For this review, take the finished solid that the model builds, in its own axes (mm). A direction names the side the tool comes from. Give positions to 0.01 mm unless a question says otherwise; leave off trailing zeros. Loops run counter-clockwise (first coordinate to the right, second up) from the corner with the lowest first, then second, coordinate; pieces in that order, holes last.
```python
from build123d import *

# Parameters (mm, degrees)
BOSS_EXTRUDE1_DEPTH = 6.2
BOSS_EXTRUDE1_DRAFT = 6
SKETCH2_R           = 1.5
SKETCH2_R_2         = 2.5
CUT_EXTRUDE1_DEPTH  = 19.269236809
SHELL1_T            = -1.2


with BuildPart() as part:
    # Sketch1 → Boss-Extrude1 (with draft: the straight prism first)
    with BuildSketch(Plane(origin=(0, 0, 0), x_dir=(1, 0, 0), z_dir=(0, 1, 0))):
        with BuildLine():
            Line((-11.5, 11.5), (-11.5, 0))
            ThreePointArc((-11.5, 0), (0, -11.5), (11.5, 0))
            Line((11.5, 0), (11.5, 11.5))
            Line((11.5, 11.5), (-11.5, 11.5))
        make_face()
    extrude(amount=-BOSS_EXTRUDE1_DEPTH)
    # Boss-Extrude1: the draft: its side faces are tilted about the plane it starts from
    boss_extrude1_sides = [part.faces().sort_by_distance(p)[0] for p in [
        (11.5, -3.1, -5.75),
        (0, -3.1, -11.5),
        (-11.5, -3.1, -5.75),
        (0, -3.1, 11.5),
    ]]
    draft(boss_extrude1_sides, Plane(origin=(0, 0, 0), x_dir=(1, 0, 0), z_dir=(0, 1, 0)), BOSS_EXTRUDE1_DRAFT)

    # Sketch2 → Cut-Extrude1 (cut, through all)
    with BuildSketch(Plane(origin=(0, 0, 0), x_dir=(1, 0, 0), z_dir=(0, 1, 0))):
        with Locations(Location((-6, 3.464101615, 0), (0, 0, 270))):
            Circle(SKETCH2_R)
        with Locations(Location((6, 3.464101615, 0), (0, 0, 270))):
            Circle(SKETCH2_R)
        with Locations(Location((0, -6.92820323, 0), (0, 0, 270))):
            Circle(SKETCH2_R_2)
    extrude(amount=-CUT_EXTRUDE1_DEPTH, mode=Mode.SUBTRACT)

    # Shell1
    shell1_openings = [part.faces().sort_by_distance(p)[0] for p in [
        (0, -6.2, -1.388400602),
    ]]
    offset(amount=SHELL1_T, openings=shell1_openings)


solid = part.part
```
Q1. For probe 1 along Z at (x, y) = (-6.25, -4.5); probe 2 along Z at (x, y) = (8, -3.5); probe 3 along Z at (x, y) = (-3, -3.75), list the stretches that pass through material, from the lowest coordinate up.
Answers:
probe 1: z = -11.97 to -10.77, -6.15 to -4.94, -1.99 to -0.78, 8.77 to 10.21
probe 2: z = -11.87 to -10.66, -5.28 to -1.65, 7.05 to 8.77
probe 3: z = -11.89 to -10.69, 4.76 to 9.09, 10.26 to 11.51
Q2. Consider section B-B on x = 0. Give the boundary of the cut face in (y, z), plus the area to 3 significant figures.
Answers:
outline: (-6.2, -12.15) - (0, -11.5) - (0, 4.43) - (-6.2, 4.43) - (-6.2, 3.23) - (-1.2, 3.23) - (-1.2, -10.42) - (-6.2, -10.95) - close; (-6.2, 9.43) - (0, 9.43) - (0, 11.5) - (-6.2, 12.15) - (-6.2, 10.95) - (-3.19, 10.63) - (-6.2, 10.63) - close
area: 45.6 mm2
Q3. Machinability: for faces 1 (the cylindrical face through (6.451, -3.057, -2.033)), 2 (the flat face through (0.15, -3.67, -10.68)), which of the approach directions +Z, -Z, +X, -X, +Y, -Y give a long, thin tool a straight path to every point of the face, cutting with its end or side? Answer none if there is none.
Answers:
face 1: +Y, -Y
face 2: -Y
Q4. Mouldability with a two-part tool opening along Z and no side actions: class faces 3 (the flat face through (10.68, -3.67, -5.4)), 4 (the conical face through (-0.258, -2.368, 11.746)), 5 (the flat face through (0, -6.2, 4)) as +Z half, -Z half, draft (parallel to the pull), parting line (faces both ways), or undercut.
Answers:
face 3: undercut
face 4: +Z half
face 5: draft
Q5. Consider section A-A on y = -2.75. Give the boundary of the cut face in (x, z), plus the area to 3 significant figures.
Answers:
outline: (-11.79, -11.79) - (11.79, -11.79) - (11.79, 0) arc R11.79 ccw to (-11.79, 0) - close; circle Ø5.4 at (-6, -3.46); circle Ø5.4 at (6, -3.46); hole (-10.58, -10.58) - (10.58, -10.58) - (10.58, 0) arc R10.58 ccw to (0.72, 10.56) arc R3.7 cw (long way) to (-0.72, 10.56) arc R10.58 ccw to (-10.58, 0) - close; hole circle Ø3 at (-6, -3.46); hole circle Ø5 at (0, 6.93); hole circle Ø3 at (6, -3.46)
area: 151 mm2
Q6. Consider section D-D on z = -7.25. Give the boundary of the cut face in (x, y).
Answers:
outline: (-12.15, -6.2) - (-10.95, -6.2) - (-10.42, -1.2) - (10.42, -1.2) - (10.95, -6.2) - (12.15, -6.2) - (11.5, 0) - (-11.5, 0) - close
Q7. Consider section C-C on y = -5.5. Give the boundary of the cut face in (x, z), plus the area to 3 significant figures.
Answers:
outline: (-12.08, -12.08) - (12.08, -12.08) - (12.08, 0) arc R12.08 ccw to (-12.08, 0) - close; circle Ø5.4 at (-6, -3.46); circle Ø7.4 at (0, 6.93); circle Ø5.4 at (6, -3.46); hole (-10.87, -10.87) - (10.87, -10.87) - (10.87, 0) arc R10.87 ccw to (-10.87, 0) - close; hole circle Ø3 at (-6, -3.46); hole circle Ø5 at (0, 6.93); hole circle Ø3 at (6, -3.46)
area: 154 mm2
Q8. For pin 1 Ø2 at (y, z) = (-4, -7) entering from +X; pin 2 Ø1.5 at (y, z) = (-2, 5.5) entering from +X, all flat-tipped, find the tip position at first contact; note any pin that passes through.
Answers:
pin 1: stops at x = 12.03
pin 2: stops at x = 10.71
